Can you work these out from the model? Positions are in its coordinate system, mm. Face numbers are marked on the shaded views. Give positions to 0.01 mm unless a question says otherwise; leave off trailing zeros. Order: outer loops, then holes, each group sorted by start corner. A loop starts at its lowest first (then second) coordinate and runs counter-clockwise, first axis right, second up. Notation, with made-up numbers: (-29.75, 57) - (29.25, 57) arc R29 ccw to (29.25, 90) - close; hole circle Ø7 at (42, -28). An arc over 180 degrees is marked (long way). One line per question, with ' | ' between items.
```python
from build123d import *

# Parameters (mm, degrees)
PARED_START                    = -27.85
SK_PARED_W                     = 50
SK_PARED_H                     = 63.3
PARED_DEPTH                    = 6.35
CABEZA_START                   = -27.85
SK_CABEZA_R                    = 25
CABEZA_DEPTH                   = 6.35
ASIENTO_1MM_START              = -21.5
SK_ASIENTO_1MM_R               = 24
SK_ASIENTO_1MM_R_2             = 15
ASIENTO_1MM_DEPTH              = 1
PASO_CENTRAL_START             = -27.85
SK_PASO_CENTRAL_R              = 8
PASO_CENTRAL_DEPTH             = 7.35
PASANTES_M2_5_ESTATOR_J5_START = -27.85
SK_PASANTES_M2_5_ESTATOR_J5_R  = 1.45
PASANTES_M2_5_ESTATOR_J5_DEPTH = 7.35
CAJAS_M2_5_J5_START            = -27.85
SK_CAJAS_M2_5_J5_R             = 2.75
CAJAS_M2_5_J5_DEPTH            = 2.5
SK_ROSCA_M3_DESDE_ABAJO_R      = 1.25
ROSCA_M3_DESDE_ABAJO_DEPTH     = 9


with BuildPart() as part:
    # Sk_Pared → Pared (new body)
    with BuildSketch(Plane(origin=(0, 0, 0), x_dir=(1, 0, 0), z_dir=(0, 1, 0)).offset(PARED_START)):
        with Locations((0, -458)):
            Rectangle(SK_PARED_W, SK_PARED_H)
    extrude(amount=PARED_DEPTH)

    # Sk_Cabeza → Cabeza (add)
    with BuildSketch(Plane(origin=(0, 0, 0), x_dir=(1, 0, 0), z_dir=(0, 1, 0)).offset(CABEZA_START)):
        with Locations((0, -490)):
            Circle(SK_CABEZA_R)
    extrude(amount=CABEZA_DEPTH)

    # Sk_Asiento_1mm → Asiento_1mm (add)
    with BuildSketch(Plane(origin=(0, 0, 0), x_dir=(1, 0, 0), z_dir=(0, 1, 0)).offset(ASIENTO_1MM_START)):
        with Locations(Location((0, -490, 0), (0, 0, 90))):
            Circle(SK_ASIENTO_1MM_R)
        with Locations(Location((0, -490, 0), (0, 0, 270))):
            Circle(SK_ASIENTO_1MM_R_2, mode=Mode.SUBTRACT)
    extrude(amount=ASIENTO_1MM_DEPTH)

    # Sk_Paso_central → Paso_central (cut)
    with BuildSketch(Plane(origin=(0, 0, 0), x_dir=(1, 0, 0), z_dir=(0, 1, 0)).offset(PASO_CENTRAL_START)):
        with Locations(Location((0, -490, 0), (0, 0, 90))):
            Circle(SK_PASO_CENTRAL_R)
    extrude(amount=PASO_CENTRAL_DEPTH, mode=Mode.SUBTRACT)

    # Sk_Pasantes_M2-5_estator_J5 → Pasantes_M2-5_estator_J5 (cut)
    with BuildSketch(Plane(origin=(0, 0, 0), x_dir=(1, 0, 0), z_dir=(0, 1, 0)).offset(PASANTES_M2_5_ESTATOR_J5_START)):
        with Locations(Location((20.5, -490, 0), (0, 0, 270))):
            Circle(SK_PASANTES_M2_5_ESTATOR_J5_R)
        with Locations(Location((10.25, -507.753520778, 0), (0, 0, 270))):
            Circle(SK_PASANTES_M2_5_ESTATOR_J5_R)
        with Locations(Location((-10.25, -507.753520778, 0), (0, 0, 270))):
            Circle(SK_PASANTES_M2_5_ESTATOR_J5_R)
        with Locations(Location((-20.5, -490, 0), (0, 0, 270))):
            Circle(SK_PASANTES_M2_5_ESTATOR_J5_R)
        with Locations(Location((-10.25, -472.246479222, 0), (0, 0, 270))):
            Circle(SK_PASANTES_M2_5_ESTATOR_J5_R)
        with Locations(Location((10.25, -472.246479222, 0), (0, 0, 270))):
            Circle(SK_PASANTES_M2_5_ESTATOR_J5_R)
    extrude(amount=PASANTES_M2_5_ESTATOR_J5_DEPTH, mode=Mode.SUBTRACT)

    # Sk_Cajas_M2-5_J5 → Cajas_M2-5_J5 (cut)
    with BuildSketch(Plane(origin=(0, 0, 0), x_dir=(1, 0, 0), z_dir=(0, 1, 0)).offset(CAJAS_M2_5_J5_START)):
        with Locations(Location((10.25, -507.753520778, 0), (0, 0, 270))):
            Circle(SK_CAJAS_M2_5_J5_R)
        with Locations(Location((-10.25, -507.753520778, 0), (0, 0, 270))):
            Circle(SK_CAJAS_M2_5_J5_R)
        with Locations(Location((-10.25, -472.246479222, 0), (0, 0, 270))):
            Circle(SK_CAJAS_M2_5_J5_R)
        with Locations(Location((10.25, -472.246479222, 0), (0, 0, 270))):
            Circle(SK_CAJAS_M2_5_J5_R)
    extrude(amount=CAJAS_M2_5_J5_DEPTH, mode=Mode.SUBTRACT)

    # Sk_Rosca_M3_desde_abajo → Rosca_M3_desde_abajo (cut)
    with BuildSketch(Plane(origin=(0, 0, 426.35), x_dir=(-1, 0, 0), z_dir=(0, 0, -1))):
        with Locations((15, -24.675)):
            Circle(SK_ROSCA_M3_DESDE_ABAJO_R)
        with Locations((-15, -24.675)):
            Circle(SK_ROSCA_M3_DESDE_ABAJO_R)
    extrude(amount=-ROSCA_M3_DESDE_ABAJO_DEPTH, mode=Mode.SUBTRACT)


solid = part.part
```
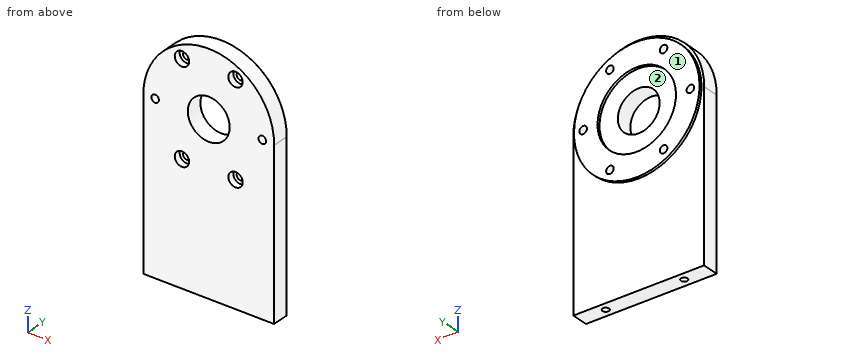
(1) Imagine slicing it at A-A (x = 0). List the corners of the cut face in (y, z) for me, and give its area (3 significant figures).
Answer below:
outline: (-27.85, 426.35) - (-21.5, 426.35) - (-21.5, 466) - (-20.5, 466) - (-20.5, 475) - (-21.5, 475) - (-21.5, 482) - (-27.85, 482) - close; (-27.85, 498) - (-21.5, 498) - (-21.5, 505) - (-20.5, 505) - (-20.5, 514) - (-21.5, 514) - (-21.5, 515) - (-27.85, 515) - close | area: 479 mm^2
(2) Imagine slicing it at D-D (x = -20.5). List the corners of the cut face in (y, z) for me, and give its area (3 significant figures).
Answer below:
outline: (-27.85, 426.35) - (-21.5, 426.35) - (-21.5, 477.52) - (-20.5, 477.52) - (-20.5, 488.55) - (-27.85, 488.55) - close; (-27.85, 491.45) - (-20.5, 491.45) - (-20.5, 502.48) - (-21.5, 502.48) - (-21.5, 504.31) - (-27.85, 504.31) - close | area: 499 mm^2
(3) If we mould it in two halves opening along X, with no side actions, what happens to the marked faces 1 and 2? For each: released by +X, released by -X, zero draft, split by the parting line, or undercut.
Answer below:
face 1: zero draft | face 2: undercut
(4) Imagine slicing it at B-B (x = 10.25). List the corners of the cut face in (y, z) for me.
Answer below:
outline: (-27.85, 426.35) - (-21.5, 426.35) - (-21.5, 468.3) - (-20.5, 468.3) - (-20.5, 470.8) - (-25.35, 470.8) - (-25.35, 469.5) - (-27.85, 469.5) - close; (-27.85, 475) - (-25.35, 475) - (-25.35, 473.7) - (-20.5, 473.7) - (-20.5, 479.05) - (-21.5, 479.05) - (-21.5, 500.95) - (-20.5, 500.95) - (-20.5, 506.3) - (-25.35, 506.3) - (-25.35, 505) - (-27.85, 505) - close; (-27.85, 510.5) - (-25.35, 510.5) - (-25.35, 509.2) - (-20.5, 509.2) - (-20.5, 511.7) - (-21.5, 511.7) - (-21.5, 512.8) - (-27.85, 512.8) - close
(5) Imagine slicing it at C-C (z = 465). List the corners of the cut face in (x, y) for me.
Answer below:
outline: (-25, -27.85) - (25, -27.85) - (25, -21.5) - (-25, -21.5) - close
(6) Will these pins go through, and if not, where does the flat tip stop? pin 1 (9 mm diameter, centred on x = 10.25, z = 507.75, fed in from +Y); pin 2 (1 mm diameter, centred on x = -5, y = -23.5, fed in from +Z); pin 3 (4 mm diameter, centred on x = -13, y = -21.5, fed in from +Z); pin 4 (2 mm diameter, centred on x = 15, y = -24.675, fed in from +Z).
Answer below:
pin 1: y = -20.5 | pin 2: z = 514.59 | pin 3: z = 512.45 | pin 4: z = 510.71
(7) If I drill on line 1 (X direction, y = -21.1, z = 490); line 2 (X direction, y = -23, z = 490); line 3 (X direction, y = -20.75, z = 507), over which ranges is the centre line in solid material (lowest first)?
Answer below:
line 1: -24 to -21.95, -19.05 to -15, 15 to 19.05, 21.95 to 24 | line 2: -25 to -21.95, -19.05 to -8, 8 to 19.05, 21.95 to 25 | line 3: -16.94 to -11.49, -9.01 to 9.01, 11.49 to 16.94
